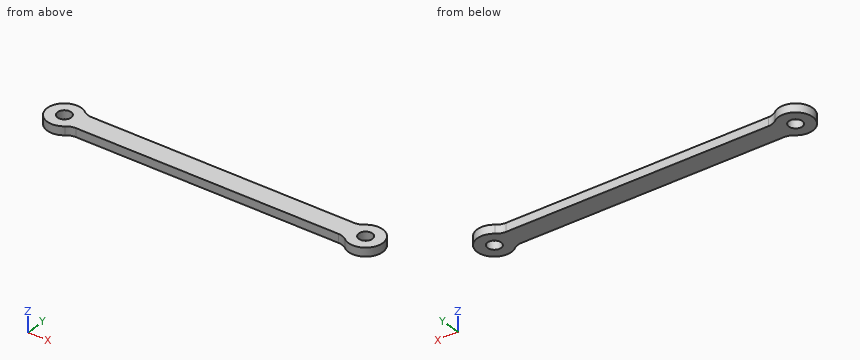
from build123d import *

# Parameters (mm, degrees)
SKETCH_1_R          = 2.1
EXTRUDE_1_DEPTH     = 5
SKETCH_2_R          = 10
EXTRUDE_2_DEPTH     = 5
SKETCH_3_R          = 4
CUT_EXTRUDE_1_DEPTH = 5
FILLET_1_R          = 8


with BuildPart() as part:
    # 草图1 → 凸台-拉伸1 (new body)
    with BuildSketch(Plane.XY):
        with BuildLine():
            Line((-88, 6), (88, 6))
            ThreePointArc((88, 6), (94, 0), (88, -6))
            Line((88, -6), (-88, -6))
            ThreePointArc((-88, -6), (-94, 0), (-88, 6))
        make_face()
        with Locations((88, 0)):
            Circle(SKETCH_1_R, mode=Mode.SUBTRACT)
        with Locations((-88, 0)):
            Circle(SKETCH_1_R, mode=Mode.SUBTRACT)
    extrude(amount=EXTRUDE_1_DEPTH)

    # 草图2 → 凸台-拉伸2 (add)
    with BuildSketch(Plane.XY.offset(5)):
        with Locations((-88, 0)):
            Circle(SKETCH_2_R)
        with Locations((88, 0)):
            Circle(SKETCH_2_R)
    extrude(amount=-EXTRUDE_2_DEPTH)

    # 草图3 → 切除-拉伸1 (cut)
    with BuildSketch(Plane.XY.offset(5)):
        with Locations((-88, 0)):
            Circle(SKETCH_3_R)
        with Locations((88, 0)):
            Circle(SKETCH_3_R)
    extrude(amount=-CUT_EXTRUDE_1_DEPTH, mode=Mode.SUBTRACT)

    # 圆角1
    fillet_1_edges = [part.edges().sort_by_distance(p)[0] for p in [
        (-80, 6, 2.5),
        (-80, -6, 2.5),
        (80, 6, 2.5),
        (80, -6, 2.5),
    ]]
    fillet(fillet_1_edges, radius=FILLET_1_R)


solid = part.part
Geometry: final body of the model. Coordinates: model frame, mm. Round coordinates to 2 decimals unless told otherwise and drop trailing zeros. Loops run counter-clockwise (first coordinate to the right, second up) from the corner with the lowest first, then second, coordinate; pieces in that order, holes last. Notation, with made-up numbers: (-31, 10) -> (8, 10) arc R35 cw to (8, 47) -> close; hole circle Ø10 at (71, -33). An arc over 180 degrees is marked (long way). One line per question, with ' | ' between items. Start each with the question number.
1. Section B-B on z = 3.8. Output: boundary loops of the cut face in (x, y), and give its area (3 significant figures).
2. Section A-A on y = 0. Output: boundary loops of the cut face in (x, z), and give its area (3 significant figures).
3. Section D-D on x = -43.5. Output: boundary loops of the cut face in (y, z).
4. Contact query for flat-ended pins moving along their axis: pin 1 (2 mm diameter, centred on y = -7.5, z = 3, fed in from +X); pin 2 (1 mm diameter, centred on x = 76, z = 1, fed in from +Y); pin 3 (1 mm diameter, centred on y = 3.5, z = 4, fed in from +X). Output: stop coordinate, or through.
5. Section C-C on x = -88. Output: boundary loops of the cut face in (y, z).
6. Line query: line 1 along Y through (x, z) = (-88, 1.2); line 2 along X through (y, z) = (1.75, 0.5); line 3 along Y through (x, z) = (64, 2.3). Output: solid intervals per line, ascending. Write a range as [from, to].
Returned:
1) outline: (-81.71, -7.78) arc R8 cw to (-76.69, -6) -> (76.69, -6) arc R8 cw to (81.71, -7.78) arc R10 ccw (long way) to (81.71, 7.78) arc R8 cw to (76.69, 6) -> (-76.69, 6) arc R8 cw to (-81.71, 7.78) arc R10 ccw (long way) to start; hole circle Ø8 at (-88, 0); hole circle Ø8 at (88, 0) | area: 2,420 mm2
2) outline: (-98, 0) -> (-92, 0) -> (-92, 5) -> (-98, 5) -> close; (-84, 0) -> (84, 0) -> (84, 5) -> (-84, 5) -> close; (92, 0) -> (98, 0) -> (98, 5) -> (92, 5) -> close | area: 900 mm2
3) outline: (-6, 0) -> (6, 0) -> (6, 5) -> (-6, 5) -> close
4) pin 1: stops at x = 95.6 | pin 2: stops at y = 6 | pin 3: stops at x = 97.54
5) outline: (-10, 0) -> (-4, 0) -> (-4, 5) -> (-10, 5) -> close; (4, 0) -> (10, 0) -> (10, 5) -> (4, 5) -> close
6) line 1: y = [-10, -4], [4, 10] | line 2: x = [-97.85, -91.6], [-84.4, 84.4], [91.6, 97.85] | line 3: y = [-6, 6]
